```python
from build123d import *

# Parameters (mm, degrees)
BOSS_EXTRUDE1_DEPTH = 76.2
BOSS_EXTRUDE2_DEPTH = 12.7
SKETCH3_R           = 15.875
CUT_EXTRUDE1_DEPTH  = 298.095864158
SKETCH4_R           = 9.525
CUT_EXTRUDE2_DEPTH  = 288.998927949


with BuildPart() as part:
    # Sketch1 → Boss-Extrude1 (new body)
    with BuildSketch(Plane.XY):
        Polygon((0, 0), (69.85, 0), (69.85, -19.05), (88.9, -19.05), (88.9, 0), (184.15, 0), (184.15, -19.05), (203.2, -19.05), (203.2, 0), (273.05, 0), (273.05, 19.05), (174.625, 19.05), (174.625, 69.85), (98.425, 69.85), (98.425, 19.05), (0, 19.05), align=None)
    extrude(amount=-BOSS_EXTRUDE1_DEPTH)

    # Sketch2 → Boss-Extrude2 (add)
    with BuildSketch(Plane(origin=(0, 0, -76.2), x_dir=(-1, 0, 0), z_dir=(0, 0, -1))):
        Polygon((-98.425, 69.85), (0, 19.05), (-98.425, 19.05), align=None)
        Polygon((-273.05, 19.05), (-174.625, 69.85), (-174.625, 19.05), align=None)
    extrude(amount=-BOSS_EXTRUDE2_DEPTH)

    # Sketch3 → Cut-Extrude1 (cut, through all)
    with BuildSketch(Plane(origin=(0, 69.85, 0), x_dir=(1, 0, 0), z_dir=(0, 1, 0))):
        with Locations(Location((136.525, 38.1, 0), (0, 0, 180))):
            Circle(SKETCH3_R)
    extrude(amount=-CUT_EXTRUDE1_DEPTH, mode=Mode.SUBTRACT)

    # Sketch4 → Cut-Extrude2 (cut, through all)
    with BuildSketch(Plane(origin=(0, 19.05, 0), x_dir=(1, 0, 0), z_dir=(0, 1, 0))):
        with Locations(Location((234.95, 38.1, 0), (0, 0, 270))):
            Circle(SKETCH4_R)
        with Locations(Location((38.1, 38.1, 0), (0, 0, 270))):
            Circle(SKETCH4_R)
    extrude(amount=-CUT_EXTRUDE2_DEPTH, mode=Mode.SUBTRACT)


solid = part.part
```
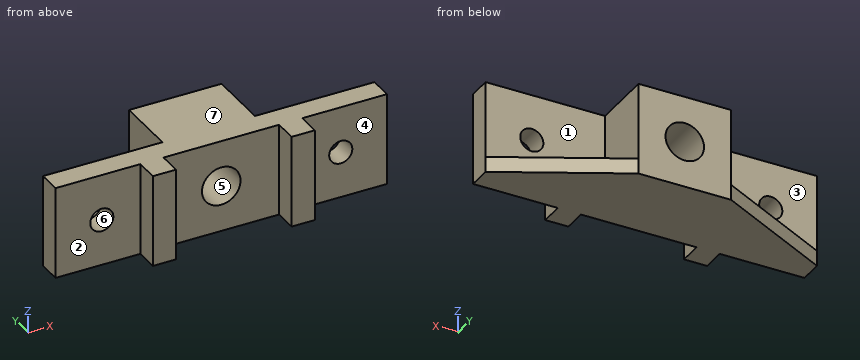
Geometry: final body of the model. Coordinates: model frame, mm. Face numbers are marked on the shaded views. A direction names the side the tool comes from. Coordinates: 2 decimals unless noted, no trailing zeros. Loops run counter-clockwise (first coordinate to the right, second up) from the corner with the lowest first, then second, coordinate; pieces in that order, holes last. Notation, with made-up numbers: (14, 89.5) -> (40, 89.5) arc R38 cw to (40, 128.5) -> close; hole circle Ø11 at (-34, 56.25). An arc over 180 degrees is marked (long way). Use a Markdown table: item, result. Add a question column.
(1) Mould query, pull axis Z, two halves, no side actions, for the marked faces 4, 5, 6 and 7. Classes: pulls with the +Z half, pulls with the -Z half, needs draft (parallel to the pull), parting line crosses it, or undercut.
(2) Access query for the marked faces 1, 2 and 3. Directions: +Z, -Z, +X, -X, +Y, -Y. A direction counts if a zero-diameter tool reaches every point of the face in a straight line with its end or side. Return the directions, or none.
(3) Section query A-A, the plane y = 16.5. Return loops of the section in (x, z) (3 decimals), plus the area to 3 significant figures.
(4) Section query D-D, the plane y = 31.5. Return loops of the section in (x, z) (3 decimals), plus the area to 3 significant figures.
(5) Pin query (flat end, axial travel): pin 1 Ø3 at (x, z) = (201.5, -30) entering from +Y; pin 2 Ø12 at (x, y) = (77, 37.5) entering from +Z; pin 3 Ø15 at (y, z) = (-11, -36) entering from +X; pin 4 Ø8 at (x, y) = (136, 23) entering from +Z. Return the tip coordinate at first contact, or that it passes through.
(6) Section query C-C, the plane x = 38.1. Return loops of the section in (y, z) (3 decimals).
(7) Line query: line 1 along X through (y, z) = (-11, -44); line 2 along X through (y, z) = (14, -38); line 3 along Z through (x, y) = (234, 4). Output: solid intervals per line, ascending.
(8) Section query B-B, the plane z = -38.1. Return loops of the section in (x, y) (3 decimals), plus the area to 3 significant figures.
Answer:
| question | item | result |
|---|---|---|
| 1 | face 4 | needs draft |
| 1 | face 5 | undercut |
| 1 | face 6 | undercut |
| 1 | face 7 | pulls with the +Z half |
| 2 | face 1 | +Z, +X, +Y |
| 2 | face 2 | +Z, -Z, -X, -Y |
| 2 | face 3 | +Z, -X, +Y |
| 3 | outline | (0, -76.2) -> (273.05, -76.2) -> (273.05, 0) -> (0, 0) -> close; hole circle Ø19.05 at (38.1, -38.1); hole circle Ø31.75 at (136.525, -38.1); hole circle Ø19.05 at (234.95, -38.1) |
| 3 | area | 19,400 mm^2 |
| 4 | outline | (24.122, -76.2) -> (248.928, -76.2) -> (248.928, -63.5) -> (174.625, -63.5) -> (174.625, 0) -> (98.425, 0) -> (98.425, -63.5) -> (24.122, -63.5) -> close; hole circle Ø31.75 at (136.525, -38.1) |
| 4 | area | 6,900 mm^2 |
| 5 | pin 1 | stops at y = 19.05 |
| 5 | pin 2 | stops at z = -63.5 |
| 5 | pin 3 | stops at x = 203.2 |
| 5 | pin 4 | stops at z = 0 |
| 6 | outline | (0, -76.2) -> (38.715, -76.2) -> (38.715, -63.5) -> (19.05, -63.5) -> (19.05, -47.625) -> (0, -47.625) -> close; (0, -28.575) -> (19.05, -28.575) -> (19.05, 0) -> (0, 0) -> close |
| 7 | line 1 | x = 69.85 to 88.9, 184.15 to 203.2 |
| 7 | line 2 | x = 0 to 28.58, 47.62 to 120.65, 152.4 to 225.43, 244.47 to 273.05 |
| 7 | line 3 | z = -76.2 to -47.58, -28.62 to 0 |
| 8 | outline | (0, 0) -> (28.575, 0) -> (28.575, 19.05) -> (0, 19.05) -> close; (47.625, 0) -> (69.85, 0) -> (69.85, -19.05) -> (88.9, -19.05) -> (88.9, 0) -> (120.65, 0) -> (120.65, 69.85) -> (98.425, 69.85) -> (98.425, 19.05) -> (47.625, 19.05) -> close; (152.4, 0) -> (184.15, 0) -> (184.15, -19.05) -> (203.2, -19.05) -> (203.2, 0) -> (225.425, 0) -> (225.425, 19.05) -> (174.625, 19.05) -> (174.625, 69.85) -> (152.4, 69.85) -> close; (244.475, 0) -> (273.05, 0) -> (273.05, 19.05) -> (244.475, 19.05) -> close |
| 8 | area | 6,850 mm^2 |
